The drawing under review shows one solid part. Ordinate dimensions are in mm from its lowest x, y, z. A direction names the side the tool comes from. Give positions to 0.01 mm unless a question says otherwise; leave off trailing zeros. Loops run counter-clockwise (first coordinate to the right, second up) from the corner with the lowest first, then second, coordinate; pieces in that order, holes last.
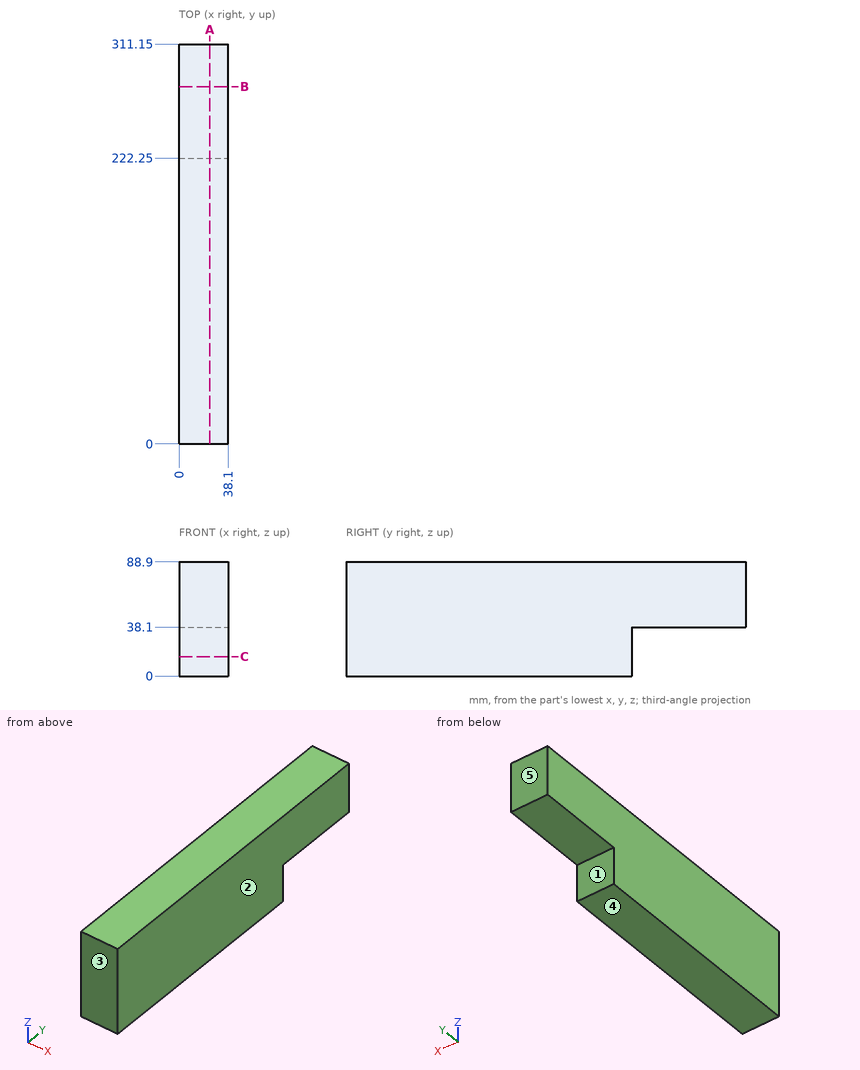
Item 1: Clearance check with flat-ended pins moving along their axes: pin 1 Ø11.5 at (x, z) = (28, 10) entering from +Y; pin 2 Ø11.5 at (x, y) = (22.5, 269.5) entering from -Z. State where each tip first meets the part, or that it passes through.
Answer:
pin 1: stops at y = 222.25
pin 2: stops at z = 38.1
Item 2: For L1, parallel to Y at x = 24.5, z = 14; L2, parallel to Z at x = 14.5, y = 235.5, list the stretches that pass through material, from the lowest coordinate up.
Answer:
L1: y = 0 to 222.25
L2: z = 38.1 to 88.9
Item 3: Take a section at B-B on y = 278. Give the boundary of the cut face in (x, z).
Answer:
outline: (0, 38.1) - (38.1, 38.1) - (38.1, 88.9) - (0, 88.9) - close
Item 4: Take a section at A-A on x = 24. Give the boundary of the cut face in (y, z), and give its area (3 significant figures).
Answer:
outline: (0, 0) - (222.25, 0) - (222.25, 38.1) - (311.15, 38.1) - (311.15, 88.9) - (0, 88.9) - close
area: 24,300 mm2
Item 5: Tool access review of the marked faces 1 and 2: name each direction out of +Z, -Z, +X, -X, +Y, -Y from which nothing blocks a thin tool from reaching the whole face with its end or side.
Answer:
face 1: -Z, +X, -X, +Y
face 2: +Z, -Z, +X, +Y, -Y
Item 6: The part is to be moulded in two halves that separate along Y. For the marked faces 3, 4 and 5, say which applies: released by +Y, released by -Y, zero draft, split by the parting line, or undercut.
Answer:
face 3: released by -Y
face 4: zero draft
face 5: released by +Y
Item 7: Take a section at C-C on z = 15. Give the boundary of the cut face in (x, y), and give its area (3 significant figures).
Answer:
outline: (0, 0) - (38.1, 0) - (38.1, 222.25) - (0, 222.25) - close
area: 8,470 mm2
